Source: CAD feature listing. Evaluate the final solid. Frame: model axes, mm. A direction names the side the tool comes from. Coordinates: 2 decimals unless noted, no trailing zeros. Write each loop counter-clockwise with the first axis right and the second up, starting at its lowest first coordinate (ties: lowest second). Pieces come first, ordered by that corner, then holes. Notation, with made-up numbers: (-0.75, 59) -> (38.25, 59) arc R28 cw to (38.25, 89) -> close; hole circle Ø5 at (-1, 80.5). An arc over 180 degrees is marked (long way). One line per item, written item: value. Start each with the question number.
1. Section query C-C, the plane y = 0.5. Output: boundary loops of the cut face in (x, z), and give its area (3 significant figures).
2. Section query A-A, the plane z = 2.25. Output: boundary loops of the cut face in (x, y).
3. Access query for faces 1 (the flat face through (7, 2, 4)), 2 (the flat face through (11, 1, 8)), 3 (the flat face through (10, 1, 7)), 4 (the flat face through (4, 7, 2)). Directions: +Z, -Z, +X, -X, +Y, -Y. A direction counts if a zero-diameter tool reaches every point of the face in a straight line with its end or side. Return the directions, or none.
4. Section query B-B, the plane x = 5.25. Output: boundary loops of the cut face in (y, z), and give its area (3 significant figures).
5. Mould query, pull axis X, two halves, no side actions, for faces 5 (the flat face through (6, 1, 6)), 6 (the flat face through (9, 7, 4)), 7 (the flat face through (2, 4, 1)). Classes: released by +X, released by -X, zero draft, split by the parting line, or undercut.
6. Section query D-D, the plane z = 7. Output: boundary loops of the cut face in (x, y), and give its area (3 significant figures).
7. Line query: line 1 (Y direction, x = 7.25, z = 3.5); line 2 (Y direction, x = 9.5, z = 5.75); line 3 (Z direction, x = 4.5, y = 1.5). Output: solid intervals per line, ascending.
8. First-contact query: P1, Ø1, axis at y = 7, z = 1, coming from the -X side; P2, Ø0.6, axis at x = 6.5, y = 7.5, coming from the +Z side; P3, Ø1, axis at x = 5.5, y = 1, coming from the +Z side. Flat tips, straight axial feed; report the tip coordinate or a pass-through.
from build123d import *

# Parameters (mm, degrees)
BOSS_EXTRUDE1_DEPTH = 8
CUT_EXTRUDE1_DEPTH  = 18
SKETCH3_W           = 7
SKETCH3_H           = 2
CUT_EXTRUDE2_DEPTH  = 2


with BuildPart() as part:
    # Sketch1 → Boss-Extrude1 (new body)
    with BuildSketch(Plane.XY):
        Polygon((0, 0), (13, 0), (13, 8), (4, 8), (4, 6), (0, 2), align=None)
    extrude(amount=BOSS_EXTRUDE1_DEPTH)

    # Sketch2 → Cut-Extrude1 (cut)
    with BuildSketch(Plane(origin=(13, 0, 0), x_dir=(0, 0, -1), z_dir=(1, 0, 0))):
        Polygon((-8, 8), (-4, 8), (-4, 6), (-2, 6), (-2, 2), (-8, 2), (-8, 6), align=None)
    extrude(amount=-CUT_EXTRUDE1_DEPTH, mode=Mode.SUBTRACT)

    # Sketch3 → Cut-Extrude2 (cut)
    with BuildSketch(Plane(origin=(0, 2, 0), x_dir=(1, 0, 0), z_dir=(0, 1, 0))):
        with Locations((6.5, -7)):
            Rectangle(SKETCH3_W, SKETCH3_H)
    extrude(amount=-CUT_EXTRUDE2_DEPTH, mode=Mode.SUBTRACT)


solid = part.part
Computed values:
1. outline: (0, 0) -> (13, 0) -> (13, 8) -> (10, 8) -> (10, 6) -> (3, 6) -> (3, 8) -> (0, 8) -> close
1. area: 90.0 mm²
2. outline: (0, 0) -> (13, 0) -> (13, 2) -> (0, 2) -> close; (4, 6) -> (13, 6) -> (13, 8) -> (4, 8) -> close
3. face 1: +Z, +X, -X
3. face 2: +Z, +X, -X, +Y, -Y
3. face 3: +Z, +Y, -Y
3. face 4: +Z, -Z, -X, +Y
4. outline: (0, 0) -> (8, 0) -> (8, 4) -> (6, 4) -> (6, 2) -> (2, 2) -> (2, 6) -> (0, 6) -> close
4. area: 28.0 mm²
5. face 5: undercut
5. face 6: zero draft
5. face 7: released by -X
6. outline: (0, 0) -> (3, 0) -> (3, 2) -> (0, 2) -> close; (10, 0) -> (13, 0) -> (13, 2) -> (10, 2) -> close
6. area: 12.0 mm²
7. line 1: y = 0 to 2, 6 to 8
7. line 2: y = 0 to 2
7. line 3: z = 0 to 6
8. P1: stops at x = 4
8. P2: stops at z = 4
8. P3: stops at z = 6
